Could you check a few things on this drawing? It's one solid part, dimensions in mm from its lowest x, y, z. A direction names the side the tool comes from. Round coordinates to 2 decimals unless told otherwise and drop trailing zeros. Order: outer loops, then holes, each group sorted by start corner. A loop starts at its lowest first (then second) coordinate and runs counter-clockwise, first axis right, second up. Notation, with made-up numbers: (-3, 14.5) - (34, 14.5) arc R14 ccw to (34, 31.5) - close; hole circle Ø8 at (-26.75, 75). An arc over 180 degrees is marked (long way). Use one line per item in the form item = value.
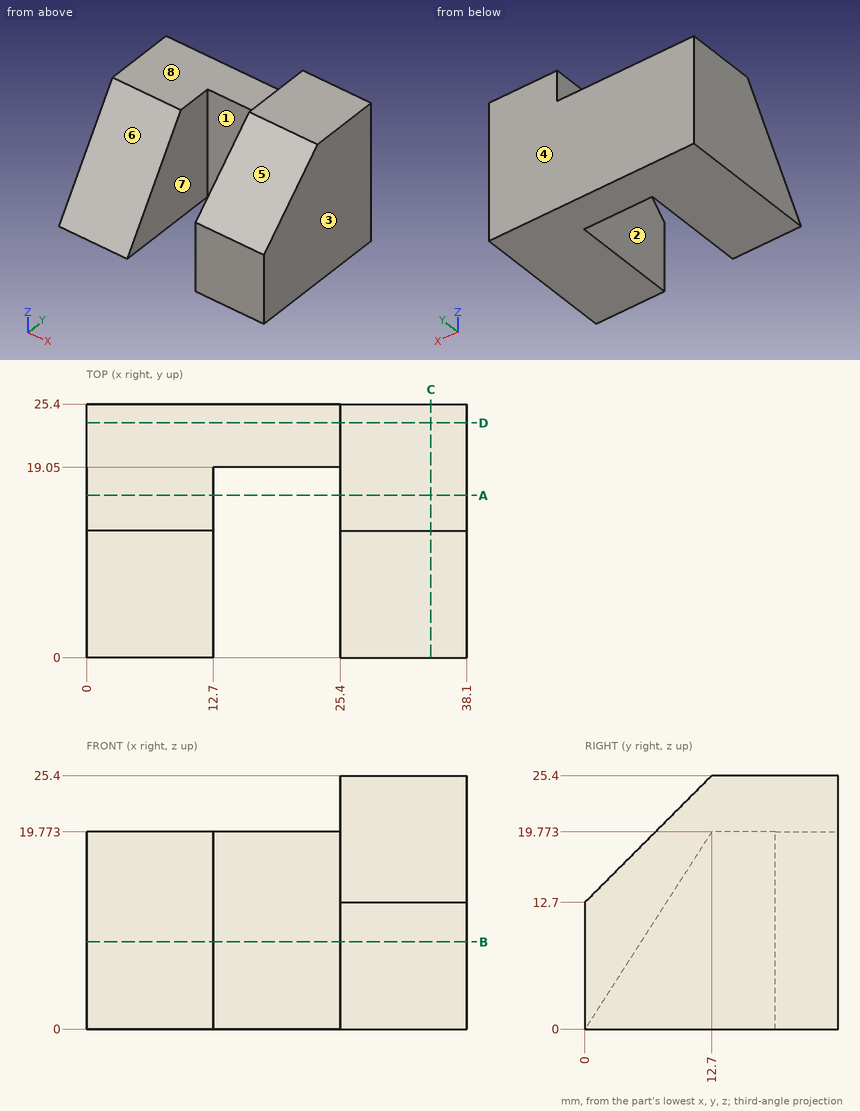
Item 1: Imagine slicing it at A-A on y = 16.25. Please give me the cut outline in (x, z).
Found:
outline = (0, 0) - (12.7, 0) - (12.7, 19.77) - (0, 19.77) - close; (25.4, 0) - (38.1, 0) - (38.1, 25.4) - (25.4, 25.4) - close
Item 2: If we mould it in two halves opening along X, with no side actions, what happens to the marked faces 1, 2, 3 and 4? For each: released by +X, released by -X, zero draft, split by the parting line, or undercut.
Found:
face_1 = undercut
face_2 = undercut
face_3 = released by +X
face_4 = zero draft
Item 3: I need wall thicknesses on L1, parallel to X at y = 9.5, z = 7; L2, parallel to X at y = 6.75, z = 12.75; L3, parallel to Y at x = 13.5, z = 19.5. Which ranges of each line are inside material? Lowest first, please.
Found:
L1 = 0 to 12.7, 25.4 to 38.1
L2 = 25.4 to 38.1
L3 = 19.05 to 25.4
Item 4: Imagine slicing it at C-C on x = 34.5. Please give me the cut outline in (y, z).
Found:
outline = (0, 0) - (25.4, 0) - (25.4, 25.4) - (12.7, 25.4) - (0, 12.7) - close
Item 5: For the marked faces 5, 6, 7 and 8, which set-ups out of +Z, -Z, +X, -X, +Y, -Y let a thin tool reach every point of the face, with its end or its side?
Found:
face_5 = +Z, +X, -X, -Y
face_6 = +Z, -X, -Y
face_7 = +Z, -Z, -Y
face_8 = +Z, -X, +Y, -Y
Item 6: Will these pins go through, and if not, where does the flat tip stop? P1, Ø4, axis at x = 22, z = 9.5, coming from the -Y side; P2, Ø4, axis at x = 17.5, y = 21.5, coming from the +Z side; P3, Ø3, axis at x = 11.5, z = 6, coming from the -Y side.
Found:
P1 = 19.05
P2 = 19.77
P3 = 2.89
Item 7: Imagine slicing it at B-B on z = 8.75. Please give me the cut outline in (x, y), plus the area to 3 significant figures.
Found:
outline = (0, 5.62) - (12.7, 5.62) - (12.7, 19.05) - (25.4, 19.05) - (25.4, 0) - (38.1, 0) - (38.1, 25.4) - (0, 25.4) - close
area = 654 mm2
Item 8: Imagine slicing it at D-D on y = 23.5. Please give me the cut outline in (x, z).
Found:
outline = (0, 0) - (38.1, 0) - (38.1, 25.4) - (25.4, 25.4) - (25.4, 19.77) - (0, 19.77) - close
